Verification items for the finished model (mm, model axes). A direction names the side the tool comes from. Round coordinates to 2 decimals unless told otherwise and drop trailing zeros. Order: outer loops, then holes, each group sorted by start corner. A loop starts at its lowest first (then second) coordinate and runs counter-clockwise, first axis right, second up. Notation, with made-up numbers: M 5.25,84.25 L 40.25,84.25 A20 ccw 40.25,121.25 Z; hole C 25.25,24.5 d7. An arc over 180 degrees is marked long. Answer as a JSON object with one key per item and string values. Group by question number.
```python
from build123d import *

# Parameters (mm, degrees)
SKETCH1_W           = 76
SKETCH1_H           = 21
BOSS_EXTRUDE1_DEPTH = 20
FILLET1_R           = 5.08
SKETCH2_R           = 1.5
CUT_EXTRUDE1_DEPTH  = 2.54


with BuildPart() as part:
    # Sketch1 → Boss-Extrude1 (new body)
    with BuildSketch(Plane(origin=(0, 0, 0), x_dir=(1, 0, 0), z_dir=(0, 1, 0))):
        Rectangle(SKETCH1_W, SKETCH1_H)
    extrude(amount=BOSS_EXTRUDE1_DEPTH)

    # Fillet1
    fillet1_edges = [part.edges().sort_by_distance(p)[0] for p in [
        (0, 20, 10.5),
        (0, 20, -10.5),
    ]]
    fillet(fillet1_edges, radius=FILLET1_R)

    # Sketch2 → Cut-Extrude1 (cut)
    with BuildSketch(Plane.XZ):
        Circle(SKETCH2_R)
    extrude(amount=-CUT_EXTRUDE1_DEPTH, mode=Mode.SUBTRACT)


solid = part.part
```
Q1. Cross-section at A-A, the plane x = 0. Record the cut outline in (y, z).
Q2. Tool access check on faces 1 (the face through (-1.5, 1.25, 0.07)), 2 (the face through (0.532, 18.472, -9.051)). Record the directions out of +Z, -Z, +X, -X, +Y, -Y that give a thin tool (end or side, any length) a straight path to the whole face; none if there is none.
Q3. Thickness scan on line 1 (Z direction, x = 0, y = 1.5); line 2 (Y direction, x = 2.5, z = -5.75); line 3 (X direction, y = 2.25, z = 1). Record the ranges inside material, lowest first. Write a range as from..to.
Q4. Release check for a two-part mould opening along Z. For faces 3 (the face through (-1, 7, -10.5)), 4 (the face through (-38, 10, 0)), 5 (the face through (0, 2.54, 0)) record: released by +Z, released by -Z, zero draft, split by the parting line, or undercut.
Q5. Cross-section at B-B, the plane z = -7.5. Record the cut outline in (x, y), then the cut area to 3 significant figures.
Q6. Cross-section at C-C, the plane x = -21. Record the cut outline in (y, z).
Q7. Gauge pin test, flat end, axial feed: pin 1 Ø0.9 at (x, z) = (0, -0.5) entering from -Y. Record the tip position at first contact, or that the pin passes through.
Conclusion:
{
 "1": {"outline": "M 0,-10.5 L 14.92,-10.5 A5.08 ccw 20,-5.42 L 20,5.42 A5.08 ccw 14.92,10.5 L 0,10.5 L 0,1.5 L 2.54,1.5 L 2.54,-1.5 L 0,-1.5 Z"},
 "2": {"face 1": "-Y", "face 2": "-Z, +X, -X, +Y"},
 "3": {"line 1": "-10.5..-1.5, 1.5..10.5", "line 2": "0..19.99", "line 3": "-38..-1.12, 1.12..38"},
 "4": {"face 3": "released by -Z", "face 4": "zero draft", "face 5": "undercut"},
 "5": {"outline": "M -38,0 L 38,0 L 38,19.55 L -38,19.55 Z", "area": "1,490 mm2"},
 "6": {"outline": "M 0,-10.5 L 14.92,-10.5 A5.08 ccw 20,-5.42 L 20,5.42 A5.08 ccw 14.92,10.5 L 0,10.5 Z"},
 "7": {"pin 1": "y = 2.54"}
}
